CAD build for the part. Positions are in the model's coordinates, mm. Face numbers are marked on the shaded views. Coordinates: 2 decimals unless noted, no trailing zeros. Loops run counter-clockwise (first coordinate to the right, second up) from the corner with the lowest first, then second, coordinate; pieces in that order, holes last. Notation, with made-up numbers: (73, -9) -> (125, -9) arc R7 cw to (125, -3) -> close; hole circle Ø1 at (-15.5, -31.5). An arc over 180 degrees is marked (long way). Write each question's results on one line, items separated by ' | '.
Autodesk Inventor part; units mm, degrees
ref_plane "YZ Plane" through (0, 0, 0) normal (1, 0, 0) x (0, 1, 0)
ref_plane "XZ Plane" through (0, 0, 0) normal (0, 1, 0) x (-1, 0, 0)
ref_plane "XY Plane" through (0, 0, 0) normal (0, 0, 1) x (1, 0, 0)
sketch "スケッチ1" plane through (0, 0, 0) normal (0, 0, 1) x (1, 0, 0)
  line L0 (4, 15.1) -> (12, 15.1)
  line L1 (12, 15.1) -> (12, -3)
  line L2 (4, -3) -> (4, 15.1)
  circle A0 centre (8, 9.7) radius 1.25
  circle A1 centre (50, 5.4) radius 1.15
  circle A2 centre (8, -5.4) radius 1.15
  circle A3 centre (50, -5.4) radius 1.15
  circle A4 centre (8, 5.4) radius 1.15
  line L3 (-1, 21.7) -> (66, 21.7)
  line L4 (-2, 20.7) -> (-2, -20.7)
  line L5 (66, -21.7) -> (-1, -21.7)
  circle A5 centre (8, 13.15) radius 0.75
  circle A6 centre (8, 0.95) radius 0.75
  line L6 (6.8, 15.1) -> (9.4, 15.1)
  line L7 (9.1, -3) -> (9.1, -1)
  line L8 (9.1, -1) -> (6.9, -1)
  line L9 (6.9, -1) -> (6.9, -3)
  circle A7 centre (8, -5.4) radius 2
  line L10 (12, -3) -> (9.1, -3)
  line L11 (6.9, -3) -> (4, -3)
  line L12 (49.4, 10.95) -> (50.6, 10.95)
  arc A8 (51.5, 10.05) -> (50.6, 10.95) centre (50.6, 10.05) ccw
  line L13 (50.6, 8.45) -> (49.4, 8.45)
  arc A9 (48.5, 9.35) -> (49.4, 8.45) centre (49.4, 9.35) ccw
  arc A10 (66, -21.7) -> (67, -20.7) centre (66, -20.7) ccw
  arc A11 (67, 20.7) -> (66, 21.7) centre (66, 20.7) ccw
  arc A12 (-1, 21.7) -> (-2, 20.7) centre (-1, 20.7) ccw
  arc A13 (-2, -20.7) -> (-1, -21.7) centre (-1, -20.7) ccw
  line L14 (9.5, -0.55) -> (3.96, -0.55)
  line L15 (3.96, -0.55) -> (3.96, 2.45)
  line L16 (3.96, 2.45) -> (9.5, 2.45)
  line L17 (9.5, 2.45) -> (9.5, -0.55)
  line L18 (9.5, 11.65) -> (3.96, 11.65)
  line L19 (3.96, 11.65) -> (3.96, 14.65)
  line L20 (3.96, 14.65) -> (9.5, 14.65)
  line L21 (9.5, 14.65) -> (9.5, 11.65)
  line L22 (54, 9) -> (67, 9)
  line L23 (67, 20.7) -> (67, 9)
  line L24 (67, -7.5) -> (67, -20.7)
  line L25 (67, -7.5) -> (54, -7.5)
  line L26 (54, -7.5) -> (54, 9)
  line L27 (51.5, 10.05) -> (51.5, 9.35)
  arc A14 (50.6, 8.45) -> (51.5, 9.35) centre (50.6, 9.35) ccw
  line L28 (48.5, 9.35) -> (48.5, 10.05)
  arc A15 (49.4, 10.95) -> (48.5, 10.05) centre (49.4, 10.05) ccw
  point P0 (0, 0)
  point P1 (8, -2.2)
  dimension "d6" = 8
  dimension "d7" = 1.5
  dimension "d8" = 1.5
  dimension "d22" = 4
  dimension "d24" = 1.2
  dimension "d25" = 11.9
  dimension "d27" = 3
  dimension "d32" = 1.1
  dimension "d33" = 1.1
  dimension "d35" = 4.3
  dimension "d36" = 3.45
  dimension "d37" = 8.75
  dimension "d38" = 4.45
extrude "押し出し1" add sketch "スケッチ1" along normal blind 1.6 contours L0 L1 L10 L7 L8 L9 L11 L2 L14 L17 L16 L18 L21 L20 | L20 L21 L18 L2 | L16 L17 L14 L2
sketch "スケッチ2" plane through (0, 0, 1.6) normal (0, 0, 1) x (1, 0, 0)
  circle A0 centre (8, 13.15) radius 0.75
  circle A1 centre (8, 0.95) radius 0.75
  circle A2 centre (8, 9.7) radius 1.25
  circle A3 centre (8, 5.4) radius 1.15
  line L0 (12, 15.1) -> (4, 15.1)
  line L1 (4, 15.1) -> (4, -3)
  line L2 (9.1, -3) -> (12, -3)
  line L3 (12, -3) -> (12, 15.1)
  circle A4 centre (5.46, 13.15) radius 0.4
  circle A5 centre (5.46, 0.95) radius 0.4
  line L4 (4, -3) -> (6.9, -3)
  line L5 (6.9, -3) -> (6.9, -1)
  line L6 (6.9, -1) -> (9.1, -1)
  line L7 (9.1, -1) -> (9.1, -3)
  point P0 (0, 0)
  dimension "d11" = 0.8
  dimension "d12" = 0.8
  dimension "d13" = 2.54
  dimension "d14" = 2.54
extrude "押し出し2" cut sketch "スケッチ2" against normal through all contours A4 | A5
fillet "フィレット1" radius 0.5 8 edges at (4, 15.1, 0.8) (4, -3, 0.8) (6.9, -3, 0.8) (6.9, -1, 0.8) (9.1, -1, 0.8) (9.1, -3, 0.8) (12, -3, 0.8) (12, 15.1, 0.8)
properties part number "HbBatteryPcb01"
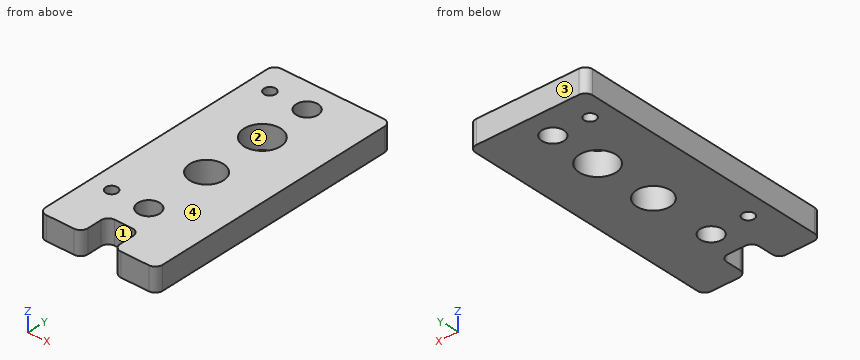
Q1. Cut at D-D on y = 5.75. Write the cut outline in (x, z), and give its area (3 significant figures).
Results are:
outline: (4, 0) -> (6.9, 0) -> (6.9, 1.6) -> (4, 1.6) -> close; (9.1, 0) -> (12, 0) -> (12, 1.6) -> (9.1, 1.6) -> close | area: 9.29 mm^2
Q2. Cut at C-C on x = 5.46. Write the cut outline in (y, z).
Results are:
outline: (-3, 0) -> (0.55, 0) -> (0.55, 1.6) -> (-3, 1.6) -> close; (1.35, 0) -> (12.75, 0) -> (12.75, 1.6) -> (1.35, 1.6) -> close; (13.55, 0) -> (15.1, 0) -> (15.1, 1.6) -> (13.55, 1.6) -> close
Q3. Pull direction Y, two halves, no side cores. Call the marked faces 1, 2, 3 and 4: +Y half, -Y half, draft (parallel to the pull), parting line (faces both ways), or undercut.
Results are:
face 1: -Y half | face 2: undercut | face 3: +Y half | face 4: draft
Q4. Wall check: L1, parallel to Y at x = 5.46, z = 1.2; L2, parallel to Y at x = 8, z = 0.3; L3, parallel to X at y = -1.75, z = 1. Give the ranges that are in metal, low to high. Write a range as from..to.
Results are:
L1: -3..0.55, 1.35..12.75, 13.55..15.1 | L2: -1..0.2, 1.7..4.25, 6.55..8.45, 10.95..12.4, 13.9..15.1 | L3: 4..6.9, 9.1..12
Q5. Cut at B-B on z = 0.5. Write the cut outline in (x, y).
Results are:
outline: (4, -2.5) arc R0.5 ccw to (4.5, -3) -> (6.4, -3) arc R0.5 ccw to (6.9, -2.5) -> (6.9, -1.5) arc R0.5 cw to (7.4, -1) -> (8.6, -1) arc R0.5 cw to (9.1, -1.5) -> (9.1, -2.5) arc R0.5 ccw to (9.6, -3) -> (11.5, -3) arc R0.5 ccw to (12, -2.5) -> (12, 14.6) arc R0.5 ccw to (11.5, 15.1) -> (4.5, 15.1) arc R0.5 ccw to (4, 14.6) -> close; hole circle Ø0.8 at (5.46, 0.95); hole circle Ø0.8 at (5.46, 13.15); hole circle Ø2.5 at (8, 9.7); hole circle Ø2.3 at (8, 5.4); hole circle Ø1.5 at (8, 0.95); hole circle Ø1.5 at (8, 13.15)
Q6. Cut at A-A on y = 13.15. Write the cut outline in (x, z), and give its area (3 significant figures).
Results are:
outline: (4, 0) -> (5.06, 0) -> (5.06, 1.6) -> (4, 1.6) -> close; (5.86, 0) -> (7.25, 0) -> (7.25, 1.6) -> (5.86, 1.6) -> close; (8.75, 0) -> (12, 0) -> (12, 1.6) -> (8.75, 1.6) -> close | area: 9.12 mm^2
